Source: CAD feature listing. Evaluate the final solid. Frame: model axes, mm. Face numbers are marked on the shaded views. Coordinates: 2 decimals unless noted, no trailing zeros. Answer as CSV lines item,"result".
Autodesk Inventor part; units mm, degrees
ref_plane "Work Plane1" through (0, -75.8, 0) normal (0, 1, 0) x (-1, 0, 0)
ref_plane "YZ Plane" through (0, 0, 0) normal (1, 0, 0) x (0, 1, 0)
ref_plane "XY Plane" through (0, 0, 0) normal (0, 0, 1) x (1, 0, 0)
sketch "Sketch1" plane through (0, 0, 0) normal (0, 1, 0) x (-1, 0, 0)
  line L0 (-51, -9.9) -> (-75.8, -9.9)
  line L1 (-75.8, -9.9) -> (-75.8, 9.9)
  line L2 (-75.8, 9.9) -> (-59.725, 9.9)
  line L3 (-59.725, 9.9) -> (-59.725, 8.8)
  line L4 (-59.725, 8.8) -> (-57.125, 9.4)
  line L5 (-57.125, 9.4) -> (-57.125, 8.2)
  line L6 (-57.125, 8.2) -> (-51, 8.2)
  line L7 (-51, 3.8) -> (-50, 3.8)
  line L8 (-50, 3.8) -> (-50, 2.8)
  line L9 (-50, 2.8) -> (-51, 2.8)
  line L10 (-51, 2.8) -> (-51, -9.9)
  line L11 (0, 17.0821) -> (0, -17.0821)
  line L12 (0, 0) -> (-89.5532, 0) construction
  line L13 (-51, 8.2) -> (-51, 3.8)
  line L14 (-65.125, 1.8471) -> (-65.125, -11.1229) construction
  point P0 (-75.8, 0)
  dimension "uA" = 151.6
  dimension "uC" = 19.8
  dimension "d4" = 1.1
  dimension "d5" = 0.5
  dimension "d6" = 2.6
  dimension "d7" = 1.7
  dimension "PCD" = 130.25
  dimension "uKnife" = 8
  dimension "uWeld" = 1
  dimension "d13" = 1
  dimension "uK" = 102
  dimension "uB" = 102
  dimension "uD" = 7.1
revolve "Revolution1" add sketch "Sketch1" angle 360 about axis through (0, 0, 17.0821) along (0, 0, -1)
sketch "Sketch2" plane through (0, 0, 9.9) normal (0, 0, 1) x (1, 0, 0)
  line L0 (0, 0) -> (0, 47.8719) construction
  line L1 (0, 0) -> (-12.7053, 63.8736) construction
  circle A0 centre (-12.7053, 63.8736) radius 4.25
  dimension "hole_diam" = 8.5
  dimension "d18" = 65.125
  dimension "bolt_angle" = 11.25
extrude "Extrusion1" cut sketch "Sketch2" against normal through all
pattern_circular "Circular Pattern1" count 16 over 360 about axis through (0, 0, -10) along (0, 0, 1) of "Extrusion1"
chamfer "Chamfer1" distance 1 angle 45 2 edges at (-75.8, 0, 9.9) (-75.8, 0, -9.9)
sketch "Sketch3" plane through (0, 0, 0) normal (0, 1, 0) x (-1, 0, 0)
  line L0 (-76.3, 0.25) -> (-75.3, 0.25)
  line L1 (-75.3, 0.25) -> (-75.3, -0.25)
  line L2 (-75.3, -0.25) -> (-76.3, -0.25)
  line L3 (-76.3, -0.25) -> (-76.3, 0.25)
  line L4 (0, 0) -> (-75.8, 0) construction
  line L5 (-75.8, -8.9) -> (-75.8, 8.9) construction
  line L6 (-75.3, 0.25) -> (-76.3, -0.25) construction
  line L7 (-76.3, 0.25) -> (-75.3, -0.25) construction
  line L8 (0, -15.82) -> (0, 15.82)
  point P0 (-75.3, 0)
  point P1 (-75.8, 0.25)
  dimension "d28" = 1
  dimension "d29" = 0.5
revolve "Revolution2" cut sketch "Sketch3" angle 360 about axis through (0, 0, -10) along (0, 0, 1)
ref_plane "Work Plane1" through (0, -75.8, 0) normal (0, 1, 0) x (-1, 0, 0)
sketch "Sketch4" plane through (0, -75.8, 0) normal (0, 1, 0) x (-1, 0, 0)
  line L0 (1, 10.9) -> (1, 8.9)
  line L1 (1, 8.9) -> (-1, 8.9)
  line L2 (-1, 8.9) -> (-1, 10.9)
  line L3 (-1, 10.9) -> (1, 10.9)
  line L4 (0, 0) -> (0, 11.6519) construction
  line L5 (-74.8, 9.9) -> (74.8, 9.9) construction
  point P0 (0, 10.9)
  point P1 (-1, 9.9)
  dimension "d31" = 2
  dimension "d32" = 2
extrude "Extrusion2" cut sketch "Sketch4" along normal up to surface
mirror "Mirror1" about plane through (0, 0, 0) normal (0, 1, 0) of "Extrusion2"
equation "\"d18\" = 0.5 * PCD"
properties part number "UFC-05" material "Stainless Steel, 440C"
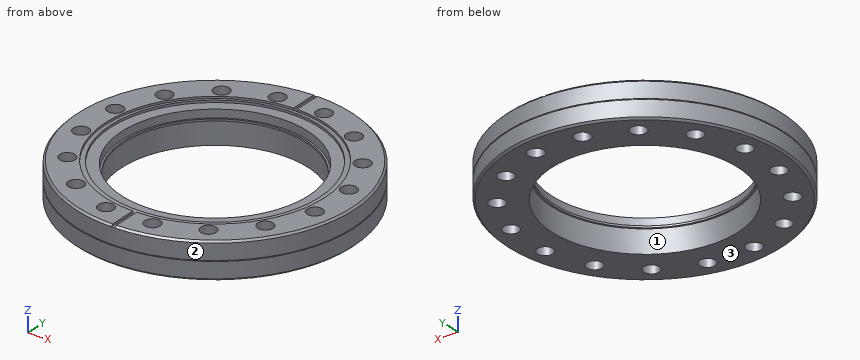
(1) Material intervals for L1, parallel to X at y = 51, z = 8.75; L2, parallel to Y at x = -65, z = 7.5; L3, parallel to X at y = 64, z = -4.75, sorted ascending. Write a range as [from, to].
Computed values:
L1,"[-56.08, -39.04], [-33.33, -25.73], [25.73, 33.33], [39.04, 56.08]"
L2,"[-39, -16.8], [-8.61, 8.61], [16.8, 39]"
L3,"[-40.62, -16.95], [-8.46, 8.46], [16.95, 40.62]"
(2) Pin query (flat end, axial travel): pin 1 Ø2 at (x, z) = (-29.5, -5.5) entering from +Y; pin 2 Ø7.5 at (x, y) = (-12.71, -63.87) entering from -Z; pin 3 Ø3 at (y, z) = (44, -7) entering from +X; pin 4 Ø4 at (y, z) = (48.5, 3) entering from -X. Return the tip coordinate at first contact, or that it passes through.
Computed values:
pin 1,"y = 70.24"
pin 2,"through"
pin 3,"x = 62.76"
pin 4,"x = -59.86"
(3) Draft query along X for the marked faces 1, 2 and 3. Return one class per face: released by +X, released by -X, zero draft, split by the parting line, or undercut.
Computed values:
face 1,"undercut"
face 2,"split by the parting line"
face 3,"zero draft"
